```python
from build123d import *

# Parameters (mm, degrees)
CROQUIS1_W              = 30
CROQUIS1_H              = 30
SALIENTE_EXTRUIR1_DEPTH = 3
CROQUIS2_W              = 3
CROQUIS2_H              = 25
SALIENTE_EXTRUIR2_DEPTH = 30
CROQUIS3_R              = 4.0394072
CORTAR_EXTRUIR1_DEPTH   = 10
CROQUIS4_W              = 22.8
CROQUIS4_H              = 22.8
CROQUIS4_W_2            = 16.8
CROQUIS4_H_2            = 16.8
SALIENTE_EXTRUIR3_DEPTH = 10


with BuildPart() as part:
    # Croquis1 → Saliente-Extruir1 (new body)
    with BuildSketch(Plane(origin=(0, 0, 0), x_dir=(1, 0, 0), z_dir=(0, 1, 0))):
        Rectangle(CROQUIS1_W, CROQUIS1_H)
    extrude(amount=SALIENTE_EXTRUIR1_DEPTH)

    # Croquis2 → Saliente-Extruir2 (add)
    with BuildSketch(Plane(origin=(0, 3, 0), x_dir=(1, 0, 0), z_dir=(0, 1, 0))):
        Rectangle(CROQUIS2_W, CROQUIS2_H)
    extrude(amount=SALIENTE_EXTRUIR2_DEPTH)

    # Croquis3 → Cortar-Extruir1 (cut)
    with BuildSketch(Plane(origin=(1.5, 0, 0), x_dir=(0, 0, -1), z_dir=(1, 0, 0))):
        with Locations((0.584677198, 25.603738422)):
            Circle(CROQUIS3_R)
    extrude(amount=-CORTAR_EXTRUIR1_DEPTH, mode=Mode.SUBTRACT)

    # Croquis4 → Saliente-Extruir3 (add)
    with BuildSketch(Plane.XZ):
        Rectangle(CROQUIS4_W, CROQUIS4_H)
        Rectangle(CROQUIS4_W_2, CROQUIS4_H_2, mode=Mode.SUBTRACT)
    extrude(amount=SALIENTE_EXTRUIR3_DEPTH)


solid = part.part
```
CAD build for the part. Positions are in the model's coordinates, mm. A direction names the side the tool comes from. Round coordinates to 2 decimals unless told otherwise and drop trailing zeros. Order: outer loops, then holes, each group sorted by start corner. A loop starts at its lowest first (then second) coordinate and runs counter-clockwise, first axis right, second up.
Item 1: Tool access for faces 4 (the face through (-11.4, -5, 0)), 5 (the face through (0, -5, -11.4)), 6 (the face through (0, -5, -8.4)): list every direction of +Z, -Z, +X, -X, +Y, -Y with a clear straight run to the whole face (end or side of a thin tool).
Item 2: Mould opens along Z. For faces 1 (the face through (8.4, -5, 0)), 2 (the face through (0, 18, -12.5)), 3 (the face through (-1.5, 18, 0)) say: pulls with the +Z half, pulls with the -Z half, needs draft (parallel to the pull), parting line crosses it, or undercut.
Item 3: Saw through at C-C on z = -1.5. Write the cut outline in (x, y), then the cut area to 3 significant figures.
Item 4: Saw through at B-B on y = 27. Write the cut outline in (x, z), then the cut area to 3 significant figures.
Item 5: Saw through at A-A on z = 7.25. Write the cut outline in (x, y).
Item 6: Pin check, flat tips, straight feed: pin 1 (2.5 mm diameter, centred on x = 0, y = 15.5, fed in from -Z); pin 2 (5 mm diameter, centred on x = 0.5, y = -3.5, fed in from +Z); pin 3 (5 mm diameter, centred on x = 2, y = 26, fed in from +Z); pin 4 (12 mm diameter, centred on x = 10, y = 26.5, fed in from +Z). Stop position of each tip, or through.
Item 7: Saw through at D-D on x = 4. Write the cut outline in (y, z), then the cut area to 3 significant figures.
Item 8: Probe line 1 along X through (y, z) = (-4, -0.75); line 2 along Y through (x, z) = (12.5, -3); line 3 along X through (y, z) = (19, -0.5). List the from-to ranges inside material, lowest first.
Reported:
1. face 4: +Z, -Z, -X, -Y
1. face 5: -Z, +X, -X, -Y
1. face 6: -Y
2. face 1: undercut
2. face 2: pulls with the -Z half
2. face 3: needs draft
3. outline: (-15, 0) - (-11.4, 0) - (-11.4, -10) - (-8.4, -10) - (-8.4, 0) - (8.4, 0) - (8.4, -10) - (11.4, -10) - (11.4, 0) - (15, 0) - (15, 3) - (1.5, 3) - (1.5, 21.67) - (-1.5, 21.67) - (-1.5, 3) - (-15, 3) - close; (-1.5, 29.54) - (1.5, 29.54) - (1.5, 33) - (-1.5, 33) - close
3. area: 216 mm2
4. outline: (-1.5, -12.5) - (1.5, -12.5) - (1.5, -4.38) - (-1.5, -4.38) - close; (-1.5, 3.21) - (1.5, 3.21) - (1.5, 12.5) - (-1.5, 12.5) - close
4. area: 52.3 mm2
5. outline: (-15, 0) - (-11.4, 0) - (-11.4, -10) - (-8.4, -10) - (-8.4, 0) - (8.4, 0) - (8.4, -10) - (11.4, -10) - (11.4, 0) - (15, 0) - (15, 3) - (1.5, 3) - (1.5, 33) - (-1.5, 33) - (-1.5, 3) - (-15, 3) - close
6. pin 1: stops at z = -12.5
6. pin 2: stops at z = 11.4
6. pin 3: stops at z = 12.5
6. pin 4: passes through
7. outline: (-10, -11.4) - (0, -11.4) - (0, -15) - (3, -15) - (3, 15) - (0, 15) - (0, 11.4) - (-10, 11.4) - (-10, 8.4) - (0, 8.4) - (0, -8.4) - (-10, -8.4) - close
7. area: 150 mm2
8. line 1: x = -11.4 to -8.4, 8.4 to 11.4
8. line 2: y = 0 to 3
8. line 3: x = -1.5 to 1.5
